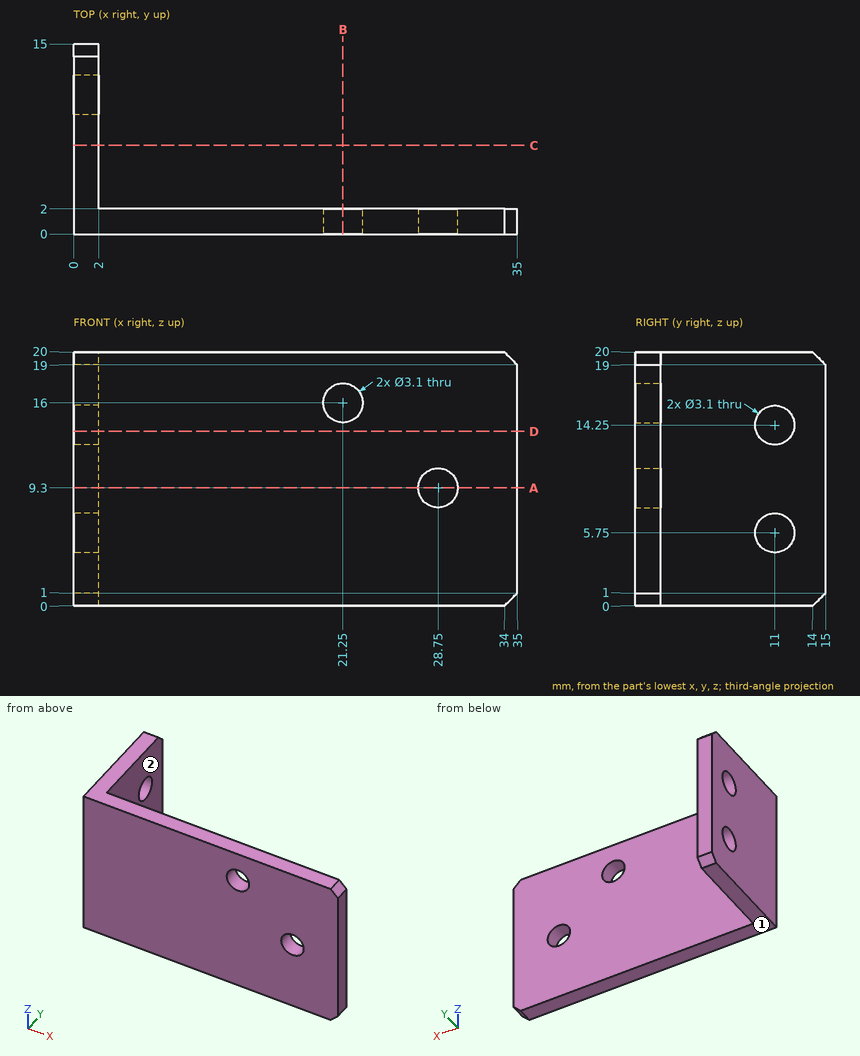
Check sheet for the drawn part. Datum: minimum x, y, z corner. Units: mm. A direction names the side the tool comes from. Coordinates: 2 decimals unless noted, no trailing zeros. Order: outer loops, then holes, each group sorted by start corner. A loop starts at its lowest first (then second) coordinate and runs counter-clockwise, first axis right, second up. Notation, with made-up numbers: M 62.5,-5.75 L 66.5,-5.75 A10 cw 66.5,11.25 Z; hole C 78.25,82 d9. An arc over 180 degrees is marked long. One line per item, written item: value. Start each with the question number.
Item 1: Access from +Z, -Z, +X, -X, +Y, -Y to the whole of each face (thin tool, end or side, straight path). Record for the marked faces 1 and 2.
Item 2: Sectioned sample at C-C (y = 7). Enter the section's corners in (x, z), then the cut area to 3 significant figures.
Item 3: Sectioned sample at B-B (x = 21.25). Enter the section's corners in (y, z), then the cut area to 3 significant figures.
Item 4: Sectioned sample at D-D (z = 13.75). Enter the section's corners in (x, y).
Item 5: Scan lines: probe 1 along Z at (x, y) = (1.35, 11); probe 2 along X at (y, z) = (3.5, 17). Record each from-to range of solid material in increasing order.
Item 6: Sectioned sample at A-A (z = 9.3). Enter the section's corners in (x, y).
Item 7: Gauge pin test, flat ends, axial feed: pin 1 (4 mm diameter, centred on y = 10.5, z = 8, fed in from +X); pin 2 (6 mm diameter, centred on x = 16, z = 10.5, fed in from -Y); pin 3 (1 mm diameter, centred on x = 24.5, z = 17.5, fed in from +Y). Record the tip position at first contact, or that the pin passes through.
Conclusion:
1. face 1: -Z, +X, -X, +Y, -Y
1. face 2: +Z, -Z, +X, +Y
2. outline: M 0,0 L 2,0 L 2,20 L 0,20 Z
2. area: 40.0 mm^2
3. outline: M 0,0 L 2,0 L 2,14.45 L 0,14.45 Z; M 0,17.55 L 2,17.55 L 2,20 L 0,20 Z
3. area: 33.8 mm^2
4. outline: M 0,0 L 35,0 L 35,2 L 2,2 L 2,9.53 L 0,9.53 Z; M 0,12.47 L 2,12.47 L 2,15 L 0,15 Z
5. probe 1: z = 0 to 4.2, 7.3 to 12.7, 15.8 to 20
5. probe 2: x = 0 to 2
6. outline: M 0,0 L 27.2,0 L 27.2,2 L 2,2 L 2,15 L 0,15 Z; M 30.3,0 L 35,0 L 35,2 L 30.3,2 Z
7. pin 1: stops at x = 2
7. pin 2: stops at y = 0
7. pin 3: stops at y = 2
